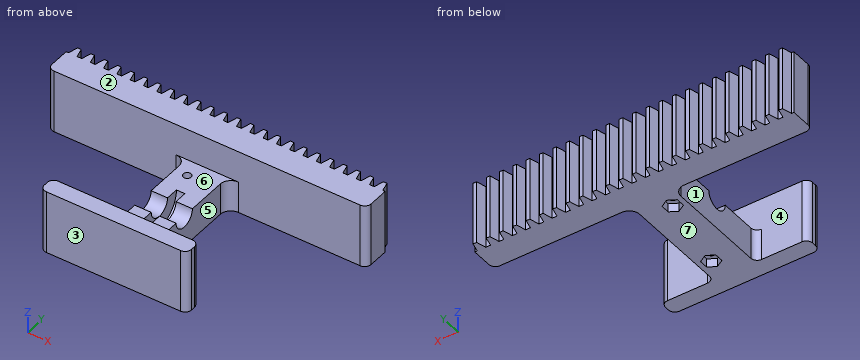
```python
from build123d import *

# Parameters (mm, degrees)
BLANKSKE_W                            = 150.8
BLANKSKE_H                            = 17
BLANK_CREMALHEIRA_DEPTH               = 30
CORTE_DENTE_DIMENSIONADO_DEPTH        = 155.692081245
CORTE_DESTES_COUNT                    = 25
CORTE_DESTES_PITCH                    = 6.2831853
SKETCH1_W                             = 9.75
SKETCH1_H                             = 55
CORPO_DE_APOIO_DEPTH                  = 30
SKETCH2_W                             = 19.5
SKETCH2_H                             = 55
REBAIXO_DEPTH                         = 15
ENCAIXE_FLANGE_11_PASSANTE_DEPTH      = 103.733441488
ENCAIXE_FLANGE_11_PASSANTE_DEPTH_BACK = 103.733441488
SKETCH3_R                             = 5.5
SKETCH3_3_R                           = 11.5
SKETCH3_3_R_2                         = 5.5
ENCAIXE_FLANGE_23X4_DEPTH             = 2
REBAIXOS_DAS_PORCAS_DEPTH             = 4
SKETCH5_R                             = 1.85
FUROS_DE_FIXA_O_DEPTH                 = 166.486071921
RAIOS_3MM_R                           = 3
RAIOS_5MM_R                           = 5


with BuildPart() as part:
    # BlankSke → Blank Cremalheira (new body)
    with BuildSketch(Plane.XY):
        with Locations((75.4, 8.5)):
            Rectangle(BLANKSKE_W, BLANKSKE_H)
    extrude(amount=-BLANK_CREMALHEIRA_DEPTH)

    # TooCutSkeSim → Corte - Dente Dimensionado (cut, through all)
    with BuildSketch(Plane.XY):
        Polygon((1.125252364, 12.5), (-1.125252364, 12.5), (-2.29560038, 17.0254), (2.29560038, 17.0254), align=None)
    corte_dente_dimensionado = extrude(amount=-CORTE_DENTE_DIMENSIONADO_DEPTH, mode=Mode.SUBTRACT)

    # Corte - Destes: Corte - Dente Dimensionado ×25
    with Locations(*[(i * CORTE_DESTES_PITCH, 0, 0) for i in range(1, CORTE_DESTES_COUNT)]):
        add(corte_dente_dimensionado, mode=Mode.SUBTRACT)

    # Sketch1 → Corpo de Apoio (add)
    with BuildSketch(Plane(origin=(0, 0, -30), x_dir=(-1, 0, 0), z_dir=(0, 0, -1))):
        with Locations((-70.525, -27.5)):
            Rectangle(SKETCH1_W, SKETCH1_H)
        with Locations((-80.275, -27.5)):
            Rectangle(SKETCH1_W, SKETCH1_H)
        Polygon((-65.65, -55), (-75.4, -55), (-75.4, -63), (-40.65, -63), (-40.65, -55), align=None)
        Polygon((-75.4, -63), (-75.4, -55), (-85.15, -55), (-110.15, -55), (-110.15, -63), align=None)
    extrude(amount=-CORPO_DE_APOIO_DEPTH)

    # Sketch2 → Rebaixo (cut)
    with BuildSketch(Plane.XY):
        with Locations((75.4, -27.5)):
            Rectangle(SKETCH2_W, SKETCH2_H)
    extrude(amount=-REBAIXO_DEPTH, mode=Mode.SUBTRACT)

    # Sketch3 → Encaixe Flange - Ø11 Passante (cut, two sides: drawn at the far end of the back side and taken through both)
    with BuildSketch(Plane.ZY.offset(-75.4).offset(-ENCAIXE_FLANGE_11_PASSANTE_DEPTH_BACK)):
        with Locations((-15, -29.25)):
            Circle(SKETCH3_R)
    extrude(amount=ENCAIXE_FLANGE_11_PASSANTE_DEPTH + ENCAIXE_FLANGE_11_PASSANTE_DEPTH_BACK, mode=Mode.SUBTRACT)

    # Sketch3<3> → Encaixe Flange - Ø23x4 (cut, symmetric)
    with BuildSketch(Plane.ZY.offset(-75.4)):
        with Locations((-15, -29.25)):
            Circle(SKETCH3_3_R)
        with Locations((-15, -29.25)):
            Circle(SKETCH3_3_R_2, mode=Mode.SUBTRACT)
    extrude(amount=ENCAIXE_FLANGE_23X4_DEPTH, both=True, mode=Mode.SUBTRACT)

    # Sketch4 → Rebaixos das Porcas (cut)
    with BuildSketch(Plane(origin=(0, 0, -30), x_dir=(-1, 0, 0), z_dir=(0, 0, -1))):
        Polygon((-71.65, -3.843078062), (-75.25, -5.921539031), (-75.25, -10.078460969), (-71.65, -12.156921938), (-68.05, -10.078460969), (-68.05, -5.921539031), align=None)
        Polygon((-79.15, -40.443072948), (-82.75, -42.521533917), (-82.75, -46.678455855), (-79.15, -48.756916824), (-75.55, -46.678455855), (-75.55, -42.521533917), align=None)
    extrude(amount=-REBAIXOS_DAS_PORCAS_DEPTH, mode=Mode.SUBTRACT)

    # Sketch5 → Furos de Fixação (cut, through all)
    with BuildSketch(Plane(origin=(0, 0, -26), x_dir=(-1, 0, 0), z_dir=(0, 0, -1))):
        with Locations((-79.15, -44.599994886)):
            Circle(SKETCH5_R)
        with Locations((-71.65, -8)):
            Circle(SKETCH5_R)
    extrude(amount=-FUROS_DE_FIXA_O_DEPTH, mode=Mode.SUBTRACT)

    # Raios 3mm
    raios_3mm_edges = [part.edges().sort_by_distance(p)[0] for p in [
        (40.65, -55, -15),
        (40.65, -63, -15),
        (110.15, -63, -15),
        (110.15, -55, -15),
        (85.15, -55, -22.5),
        (65.65, -55, -22.5),
        (150.8, 0, -15),
        (0, 0, -15),
    ]]
    fillet(raios_3mm_edges, radius=RAIOS_3MM_R)

    # Raios 5mm
    raios_5mm_edges = [part.edges().sort_by_distance(p)[0] for p in [
        (85.15, 0, -22.5),
        (65.65, 0, -22.5),
    ]]
    fillet(raios_5mm_edges, radius=RAIOS_5MM_R)


solid = part.part
```
The listing builds one solid part. Answer for the finished solid, in the listing's coordinates (mm). Face numbers are marked on the shaded views. A direction names the side the tool comes from. Give positions to 0.01 mm unless a question says otherwise; leave off trailing zeros. Loops run counter-clockwise (first coordinate to the right, second up) from the corner with the lowest first, then second, coordinate; pieces in that order, holes last. Notation, with made-up numbers: M 66,54 L 106,54 A30 ccw 106,79 Z; hole C 83,62.25 d6. An arc over 180 degrees is marked long. One line per item, written item: value.
Q1. Determine the mould class of the marked faces 1, 2, 3 and 4 for opening direction Y: +Y half, -Y half, draft (parallel to the pull), parting line (faces both ways), or undercut.
Working result:
face 1: undercut
face 2: draft
face 3: -Y half
face 4: undercut
Q2. For the marked faces 5, 6 and 7, determine the directions among +Z, -Z, +X, -X, +Y, -Y from which every point of the face is accessible in a straight line to the end or side of a thin tool.
Working result:
face 5: +Z, -Z, +X
face 6: +Z, +X, -X
face 7: -Z, +X, -X, +Y, -Y
Q3. Find the intervals of material crossed by line 1 (Y direction, x = 79.15, z = -22.75); line 2 (Y direction, x = 103, z = -25.5); line 3 (X direction, y = -29, z = -25), in increasing order. Write a range as from..to.
Working result:
line 1: y = -63..-46.45, -42.75..17
line 2: y = -63..-55, 0..17
line 3: x = 65.65..73.4, 77.4..85.15
Q4. Flat-ended cylindrical pins translate along their axes: P1, Ø0.7, axis at x = 106.5, z = -10, coming from the +Y side; P2, Ø6, axis at x = 79.5, y = -46, coming from the -Z side; P3, Ø8, axis at y = -13.5, z = -12, coming from the -X side; P4, Ø1.5, axis at y = -7.5, z = -27, coming from the +X side. Find the tip coordinate at first contact, or state that the pin passes through.
Working result:
P1: stops at y = 12.5
P2: stops at z = -30
P3: stops at x = 65.65
P4: stops at x = 85.15
Q5. A cutting plane is placed at A-A on y = -8. Determine the outline of the cut face in (x, z), then the cut area to 3 significant figures.
Working result:
outline: M 65.65,-30 L 68.05,-30 L 68.05,-26 L 69.8,-26 L 69.8,-15 L 65.65,-15 Z; M 73.5,-26 L 75.25,-26 L 75.25,-30 L 85.15,-30 L 85.15,-15 L 73.5,-15 Z
area: 223 mm^2
Q6. A cutting plane is placed at B-B on z = -16.5. Give the number of separate pieces and of enclosed holes in the cut face, then the cut area to 3 significant figures.
Working result:
separate pieces: 2
enclosed holes: 2
area: 3,550 mm^2
Q7. A cutting plane is placed at C-C on y = -29.25. Determine the outline of the cut face in (x, z).
Working result:
outline: M 65.65,-30 L 85.15,-30 L 85.15,-20.5 L 77.4,-20.5 L 77.4,-26.5 L 73.4,-26.5 L 73.4,-20.5 L 65.65,-20.5 Z
